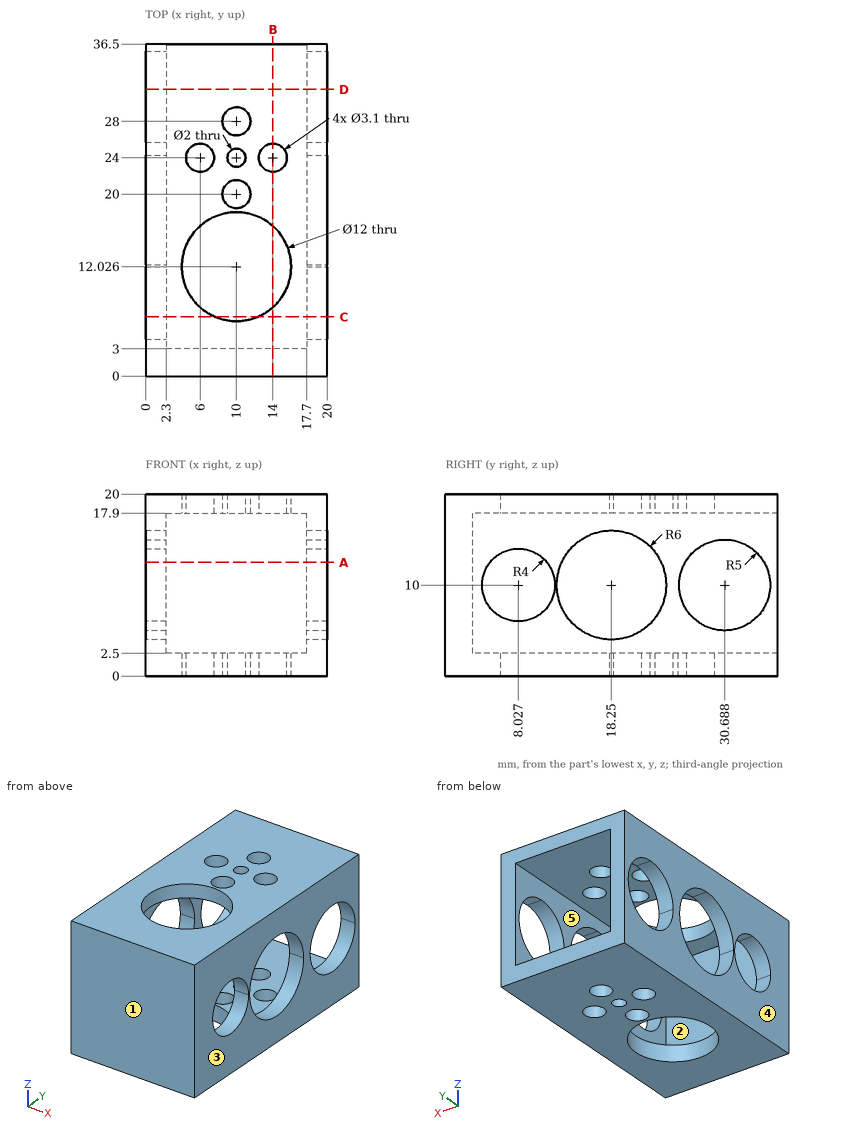
Here's the drawing with two shaded views (mm, measured from the low corner). I have some questions. A direction names the side the tool comes from. Round coordinates to 2 decimals unless told otherwise and drop trailing zeros. Loops run counter-clockwise (first coordinate to the right, second up) from the corner with the lowest first, then second, coordinate; pieces in that order, holes last.
1. Suppose I cut it at D-D, the plane y = 31.5. Please give me the cut outline in (x, z).
Answers:
outline: (0, 0) - (20, 0) - (20, 5.07) - (17.7, 5.07) - (17.7, 2.5) - (2.3, 2.5) - (2.3, 5.07) - (0, 5.07) - close; (0, 14.93) - (2.3, 14.93) - (2.3, 17.9) - (17.7, 17.9) - (17.7, 14.93) - (20, 14.93) - (20, 20) - (0, 20) - close
2. For the marked faces 1 and 2, which set-ups out of +Z, -Z, +X, -X, +Y, -Y let a thin tool reach every point of the face, with its end or its side?
Answers:
face 1: +Z, -Z, +X, -X, -Y
face 2: +Y
3. Thinking about a two-plate mould opening in X: for the marked faces 3, 4 and 5, which applies, released by +X, released by -X, zero draft, split by the parting line, or undercut?
Answers:
face 3: released by +X
face 4: released by -X
face 5: undercut
4. Suppose I cut it at B-B, the plane x = 14. Please give me the cut outline in (y, z).
Answers:
outline: (0, 0) - (7.55, 0) - (7.55, 2.5) - (3, 2.5) - (3, 17.9) - (7.55, 17.9) - (7.55, 20) - (0, 20) - close; (16.5, 0) - (22.45, 0) - (22.45, 2.5) - (16.5, 2.5) - close; (16.5, 17.9) - (22.45, 17.9) - (22.45, 20) - (16.5, 20) - close; (25.55, 0) - (36.5, 0) - (36.5, 2.5) - (25.55, 2.5) - close; (25.55, 17.9) - (36.5, 17.9) - (36.5, 20) - (25.55, 20) - close
5. If I drill on probe 1 along X at (y, z) = (24, 19.55); probe 2 along Y at (x, z) = (10, 18.85); probe 3 along Z at (x, y) = (17.5, 16), over which ranges is the centre line in solid material (lowest first)?
Answers:
probe 1: x = 0 to 4.45, 7.55 to 9, 11 to 12.45, 15.55 to 20
probe 2: y = 0 to 6.03, 18.03 to 18.45, 21.55 to 23, 25 to 26.45, 29.55 to 36.5
probe 3: z = 0 to 2.5, 17.9 to 20
6. Will these pins go through, and if not, where does the flat tip stop? pin 1 (4.5 mm diameter, centred on y = 14, z = 7, fed in from +X); pin 2 (1.9 mm diameter, centred on x = 10, y = 28, fed in from +Z); pin 3 (3 mm diameter, centred on x = 13.5, z = 5.5, fed in from +Y).
Answers:
pin 1: stops at x = 20
pin 2: passes through
pin 3: stops at y = 3
7. Suppose I cut it at A-A, the plane z = 12.5. Give the number of separate pieces and of enclosed holes in the cut face.
Answers:
separate pieces: 7
enclosed holes: 0
8. Suppose I cut it at C-C, the plane y = 6.5. Please give me the cut outline in (x, z), and give its area (3 significant figures).
Answers:
outline: (0, 0) - (7.66, 0) - (7.66, 2.5) - (2.3, 2.5) - (2.3, 6.3) - (0, 6.3) - close; (0, 13.7) - (2.3, 13.7) - (2.3, 17.9) - (7.66, 17.9) - (7.66, 20) - (0, 20) - close; (12.34, 0) - (20, 0) - (20, 6.3) - (17.7, 6.3) - (17.7, 2.5) - (12.34, 2.5) - close; (12.34, 17.9) - (17.7, 17.9) - (17.7, 13.7) - (20, 13.7) - (20, 20) - (12.34, 20) - close
area: 107 mm2
